from build123d import *

# Parameters (mm, degrees)
F1_DEPTH = 25.4
F2_DEPTH = 50.8


with BuildPart() as f1:
    # F0 (on Front) → F1 (new body)
    with BuildSketch(Plane.XZ):
        with BuildLine():
            Line((0, 0), (0, 48.2160523534))
            Line((0, 48.2160523534), (-25.3014918417, 47.261275351))
            Line((-25.3014918417, 47.261275351), (-25.3014918417, 23.7738545984))
            ThreePointArc((-25.3014918417, 23.7738545984), (-41.8645804006, 15.3146673523), (-52.4170547724, 0))
            Line((-52.4170547724, 0), (0, 0))
        make_face()
        Polygon((-25.3014918417, 47.261275351), (0, 48.2160523534), (-25.3375213031, 48.2160523534), align=None)
    extrude(amount=F1_DEPTH)

    # F2 (add): a face of the model
    f2_faces = [f1.faces().sort_by_distance(p)[0] for p in [
        (-18.7199477301, -25.4, 20.2252721756),
    ]]
    extrude(f2_faces, amount=F2_DEPTH)


solid = f1.part
Part model, mm, in its own coordinate system. Coordinates: 2 decimals unless noted, no trailing zeros. Loops run counter-clockwise (first coordinate to the right, second up) from the corner with the lowest first, then second, coordinate; pieces in that order, holes last. Notation, with made-up numbers: M 53,-25.75 L 77,-25.75 A28 ccw 77,3.25 Z; hole C 1,62 d5. An arc over 180 degrees is marked long. Use a Markdown table: item, result. Add a question column.
Q1. Probe L1, parallel to X at y = -70.5, z = 34; L2, parallel to Z at x = -48, y = -72; L3, parallel to X at y = -57.5, z = 18. List the from-to ranges inside material, lowest first.
Q2. Cut at C-C (x = -45). Write the cut outline in (y, z), and give its area (3 significant figures).
Q3. Cut at A-A (y = -24). Write the cut outline in (x, z), and give its area (3 significant figures).
Q4. Pin check, flat tips, straight feed: P1, Ø1, axis at y = -68, z = 5.5, coming from the -X side; P2, Ø1, axis at y = -40, z = 17, coming from the -X side; P3, Ø8, axis at x = -31, z = 35, coming from the -Y side. Stop position of each tip, or through.
Q5. Cut at B-B (z = 35). Write the cut outline in (x, y), and give its area (3 significant figures).
Worked out:
| question | item | result |
|---|---|---|
| 1 | L1 | x = -25.3 to 0 |
| 1 | L2 | z = 0 to 8.45 |
| 1 | L3 | x = -38.42 to 0 |
| 2 | outline | M -76.2,0 L 0,0 L 0,12.23 L -76.2,12.23 Z |
| 2 | area | 932 mm2 |
| 3 | outline | M -52.42,0 L 0,0 L 0,48.22 L -25.34,48.22 L -25.3,47.26 L -25.3,23.77 A37.94 ccw Z |
| 3 | area | 1,650 mm2 |
| 4 | P1 | stops at x = -50.13 |
| 4 | P2 | stops at x = -40.44 |
| 4 | P3 | passes through |
| 5 | outline | M -25.3,-76.2 L 0,-76.2 L 0,0 L -25.3,0 Z |
| 5 | area | 1,930 mm2 |
